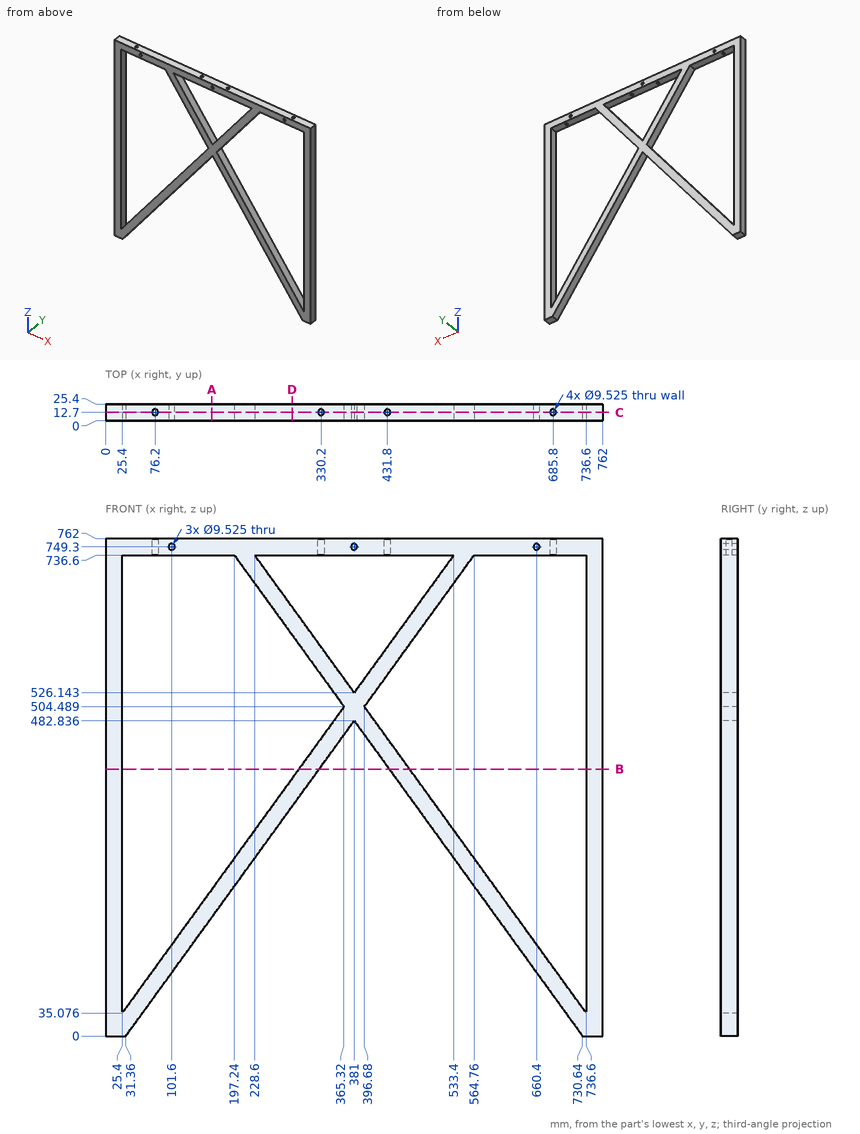
Geometry check sheet. Reference: drawing and pictorial views, mm from the part's lowest x, y, z. Round coordinates to 2 decimals unless told otherwise and drop trailing zeros. Order: outer loops, then holes, each group sorted by start corner. A loop starts at its lowest first (then second) coordinate and runs counter-clockwise, first axis right, second up. Notation, with made-up numbers: M 81,19 L 136,19 A23 cw 136,32 Z; hole C 40,36.25 d5. An arc over 180 degrees is marked long. Answer in a Markdown table with one row per item.
(1) Sectioned sample at D-D, the plane x = 286. Record the cut outline in (y, z) (1 decimal), and give its area (4 significant figures).
Responses:
| item | result |
|---|---|
| outline | M 0,351.6 L 25.4,351.6 L 25.4,395 L 0,395 Z; M 0,614 L 25.4,614 L 25.4,657.3 L 0,657.3 Z; M 0,736.6 L 25.4,736.6 L 25.4,762 L 0,762 Z |
| area | 2,845 mm² |
(2) Sectioned sample at B-B, the plane z = 409. Record the cut outline in (x, y).
Responses:
| item | result |
|---|---|
| outline | M 0,0 L 25.4,0 L 25.4,25.4 L 0,25.4 Z; M 296.17,0 L 327.53,0 L 327.53,25.4 L 296.17,25.4 Z; M 434.47,0 L 465.83,0 L 465.83,25.4 L 434.47,25.4 Z; M 736.6,0 L 762,0 L 762,25.4 L 736.6,25.4 Z |
(3) Scan lines: probe 1 along X at (y, z) = (17.75, 749.3); probe 2 along Y at (x, z) = (330.2, 750.5); probe 3 along Z at (x, y) = (381, 11.5) (1 decimal). Record each from-to range of solid material in increasing order. Write a range as from..to.
Responses:
| item | result |
|---|---|
| probe 1 | x = 0..96.84, 106.36..376.24, 385.76..655.64, 665.16..762 |
| probe 2 | y = 0..7.94, 17.46..25.4 |
| probe 3 | z = 482.8..526.1, 736.6..744.5, 754.1..762 |
(4) Go/stop test with flat-tipped pins: P1, Ø7.5, axis at x = 76.2, y = 12.7, coming from the +Z side; P2, Ø1, axis at x = 477.5, y = 13, coming from the -Z side (1 decimal); P3, Ø7.5, axis at x = 133, y = 18, coming from the -Z side; P4, Ø7.5, axis at x = 660.4, z = 749.3, coming from the -Y side. Record where each tip stops, or that it passes through.
Responses:
| item | result |
|---|---|
| P1 | stops at z = 110.41 |
| P2 | stops at z = 348.9 |
| P3 | stops at z = 135.18 |
| P4 | passes through |
(5) Sectioned sample at A-A, the plane x = 163. Record the cut outline in (y, z) (1 decimal).
Responses:
| item | result |
|---|---|
| outline | M 0,181.8 L 25.4,181.8 L 25.4,225.1 L 0,225.1 Z; M 0,736.6 L 25.4,736.6 L 25.4,762 L 0,762 Z |
(6) Sectioned sample at C-C, the plane y = 12.7. State how many separate pieces and enclosed holes the cut face has, and give its area (3 significant figures).
Responses:
| item | result |
|---|---|
| separate pieces | 2 |
| enclosed holes | 3 |
| area | 100,000 mm² |
